Can you work these out from the model? Positions are in its coordinate system, mm. A direction names the side the tool comes from. Coordinates: 2 decimals unless noted, no trailing zeros. Order: outer loops, then holes, each group sorted by start corner. A loop starts at its lowest first (then second) coordinate and runs counter-clockwise, first axis right, second up. Notation, with made-up numbers: (37.25, 62.5) - (86.25, 62.5) arc R14 cw to (86.25, 68.5) - close; hole circle Ø2 at (16, -15). An arc over 180 degrees is marked (long way). Return JSON: item names as keys, results as strings. Group by question number.
1) Imagine slicing it at C-C (x = 44). Write out the boundary of the cut face in (y, z), and give its area (3 significant figures).
2) Imagine slicing it at D-D (y = 23). Write out the boundary of the cut face in (x, z).
3) Imagine slicing it at A-A (y = 32.5). Write out the boundary of the cut face in (x, z), and give its area (3 significant figures).
4) If I drill on line 1 along X through (y, z) = (30, 31.75); line 2 along Z through (x, y) = (42.5, 15); line 3 along Y through (x, z) = (14.5, 25), over which ranges is the centre line in solid material (lowest first)?
5) Which directions (+Z, -Z, +X, -X, +Y, -Y) give clear straight access to the entire face, cutting with the end or side of a thin tool? Please do faces 1 (the face through (15, 25.4, 21)), 2 (the face through (25.4, 32, 25)), 3 (the face through (31, 15, 6.35)).
6) For pin 1 Ø5 at (x, y) = (10.5, 12) entering from +Z; pin 2 Ø11.5 at (x, z) = (12.7, 31.75) entering from +Y; pin 3 Ø12 at (y, z) = (25, 6.5) entering from -X; pin 4 Ø14 at (y, z) = (30.5, 23.5) entering from +X, each with a flat end and sliding along its axis, tell me the tip position at first contact or that it passes through.
7) Imagine slicing it at B-B (z = 32.5). Write out the boundary of the cut face in (x, y).
8) If we mould it in two halves opening along Y, with no side actions, what happens to faces 4 (the face through (51.46, 26.64, 3.13)), 5 (the face through (59.68, 3.62, 3.13)), 6 (the face through (12.979, 31.661, 44.447))? For each: pulls with the +Y half, pulls with the -Y half, needs draft (parallel to the pull), parting line crosses it, or undercut.
```python
from build123d import *

# Parameters (mm, degrees)
F0_R     = 3.175
F1_DEPTH = 6.35
F0_W     = 25.4
F0_H     = 12.7
F2_DEPTH = 31.75
F4_DEPTH = 12.7
F5_DEPTH = 12.7
F6_DEPTH = 12.7
F7_DEPTH = 6.35


with BuildPart() as f1:
    # F0 (on Top) → F1 (new body)
    with BuildSketch(Plane.XY):
        Polygon((0, 25.4), (0, 12.7), (9.525, 12.7), (12.7, 12.7), (12.7, 9.525), (12.7, 0), (50.8, 0), (50.8, 9.525), (50.8, 12.7), (53.975, 12.7), (63.5, 12.7), (63.5, 38.1), (25.4, 38.1), (25.4, 25.4), align=None)
        with Locations((53.975, 28.575)):
            Circle(F0_R, mode=Mode.SUBTRACT)
        with BuildLine():
            Line((50.8, 9.525), (50.8, 0))
            ThreePointArc((50.8, 0), (59.7802561211, 3.7197438789), (63.5, 12.7))
            Line((63.5, 12.7), (53.975, 12.7))
            ThreePointArc((53.975, 12.7), (56.2200640303, 11.7700640303), (57.15, 9.525))
            ThreePointArc((57.15, 9.525), (53.975, 6.35), (50.8, 9.525))
        make_face()
        with BuildLine():
            Line((9.525, 12.7), (0, 12.7))
            ThreePointArc((0, 12.7), (3.7197438789, 3.7197438789), (12.7, 0))
            Line((12.7, 0), (12.7, 9.525))
            ThreePointArc((12.7, 9.525), (7.2799359697, 7.2799359697), (9.525, 12.7))
        make_face()
    extrude(amount=F1_DEPTH)

    # F0 (on Top) → F2 (join)
    with BuildSketch(Plane.XY):
        with Locations((12.7, 31.75)):
            Rectangle(F0_W, F0_H)
    extrude(amount=F2_DEPTH)

    # F3 (on face) → F4 (join)
    with BuildSketch(Plane.XZ.offset(-25.4)):
        with BuildLine():
            ThreePointArc((38.1, 6.35), (29.1197438789, 10.0697438789), (25.4, 19.05))
            Line((25.4, 19.05), (25.4, 6.35))
            Line((25.4, 6.35), (38.1, 6.35))
        make_face()
    extrude(amount=-F4_DEPTH)

    # F3 (on face) → F5 (cut)
    with BuildSketch(Plane.XZ.offset(-25.4)):
        with BuildLine():
            Line((6.35, 31.75), (19.05, 31.75))
            ThreePointArc((19.05, 31.75), (12.7, 38.1), (6.35, 31.75))
        make_face()
        with BuildLine():
            ThreePointArc((6.35, 31.75), (12.7, 25.4), (19.05, 31.75))
            Line((19.05, 31.75), (6.35, 31.75))
        make_face()
    extrude(amount=-F5_DEPTH, mode=Mode.SUBTRACT)

    # F3 (on face) → F6 (join)
    with BuildSketch(Plane.XZ.offset(-25.4)):
        with BuildLine():
            Line((19.05, 31.75), (25.4, 31.75))
            ThreePointArc((25.4, 31.75), (12.7, 44.45), (0, 31.75))
            Line((0, 31.75), (6.35, 31.75))
            ThreePointArc((6.35, 31.75), (12.7, 38.1), (19.05, 31.75))
        make_face()
    extrude(amount=-F6_DEPTH)

    # F0 (on Top) → F7 (join)
    with BuildSketch(Plane.XY):
        with BuildLine():
            Line((12.7, 12.7), (9.525, 12.7))
            ThreePointArc((9.525, 12.7), (11.7700640303, 11.7700640303), (12.7, 9.525))
            Line((12.7, 9.525), (12.7, 12.7))
        make_face()
        with BuildLine():
            Line((50.8, 12.7), (50.8, 9.525))
            ThreePointArc((50.8, 9.525), (51.7299359697, 11.7700640303), (53.975, 12.7))
            Line((53.975, 12.7), (50.8, 12.7))
        make_face()
    extrude(amount=F7_DEPTH)


solid = f1.part
```
Calculated:
{
 "1": {"outline": "(0, 0) - (38.1, 0) - (38.1, 6.35) - (0, 6.35) - close", "area": "242 mm2"},
 "2": {"outline": "(0, 0) - (63.5, 0) - (63.5, 6.35) - (0, 6.35) - close"},
 "3": {"outline": "(0, 0) - (63.5, 0) - (63.5, 6.35) - (38.1, 6.35) arc R12.7 cw to (25.4, 19.05) - (25.4, 31.75) arc R12.7 ccw to (0, 31.75) - close; hole circle Ø12.7 at (12.7, 31.75)", "area": "1,210 mm2"},
 "4": {"line 1": "0 to 6.35, 19.05 to 25.4", "line 2": "0 to 6.35", "line 3": "25.4 to 38.1"},
 "5": {"face 1": "+Z, +X, -X, -Y", "face 2": "+Z, +X, +Y, -Y", "face 3": "+Z, +X, -Y"},
 "6": {"pin 1": "z = 6.35", "pin 2": "through", "pin 3": "x = 0", "pin 4": "x = 25.66"},
 "7": {"outline": "(0.02, 25.4) - (6.39, 25.4) - (6.39, 38.1) - (0.02, 38.1) - close; (19.01, 25.4) - (25.38, 25.4) - (25.38, 38.1) - (19.01, 38.1) - close"},
 "8": {"face 4": "undercut", "face 5": "pulls with the -Y half", "face 6": "needs draft"}
}
